The model under review builds one solid part; all positions refer to its coordinate system, in mm. A direction names the side the tool comes from. Coordinates: 2 decimals unless noted, no trailing zeros. Loops run counter-clockwise (first coordinate to the right, second up) from the corner with the lowest first, then second, coordinate; pieces in that order, holes last. Notation, with made-up numbers: (79.5, 5.25) - (90.5, 5.25) arc R29 ccw to (90.5, 26.25) - close; hole circle Ø5 at (5, 50.5). An arc over 180 degrees is marked (long way). Answer in a Markdown table with one row per item. Add a question column.
(1) We need section A-A on y = 26.25. Write out the cut boundary in (x, z), plus the area to 3 significant figures.
(2) For P1, Ø16.5, axis at y = 12, z = -68, coming from the -X side; P2, Ø8, axis at y = 12, z = -49, coming from the -X side; P3, Ø11, axis at x = 110, y = 21.5, coming from the +Z side, all flat-tipped, find the tip position at first contact; note any pin that passes through.
(3) For line 1 along Z through (x, y) = (135, 1.75); line 2 along Z through (x, y) = (95, 3.5); line 3 along X through (y, z) = (0.8, -70), list the stretches that pass through material, from the lowest coordinate up.
(4) We need section D-D on x = 109.5. Write out the cut boundary in (y, z), plus the area to 3 significant figures.
(5) We need section B-B on x = 135. Write out the cut boundary in (y, z), plus the area to 3 significant figures.
(6) Machinability: for faces 5 (the flat face through (12, 15, -49.271)), 6 (the flat face through (86, 10, -13)), 7 (the flat face through (47, 9, -46.789)), which of the approach directions +Z, -Z, +X, -X, +Y, -Y give a long, thin tool a straight path to every point of the face, cutting with its end or side? Answer none if there is none.
(7) Mouldability with a two-part tool opening along X and no side actions: class faces 1 (the flat face through (110, 15, -44.515)), 2 (the flat face through (7.038, 15, -44)), 3 (the flat face through (96.557, 6, -63)), 4 (the flat face through (76.557, 6, -53)) as +X half, -X half, draft (parallel to the pull), parting line (faces both ways), or undercut.
(8) We need section C-C on x = 32.5. Write out the cut boundary in (y, z), plus the area to 3 significant figures.
from build123d import *

# Parameters (mm, degrees)
ESQUISSE1_W      = 140
ESQUISSE1_H      = 75
ESQUISSE1_R      = 2
EXTRUSION1_DEPTH = 3
ESQUISSE2_W      = 45
ESQUISSE2_H      = 45
EXTRUSION2_DEPTH = 15
CONG_1_R         = 2
ESQUISSE3_W      = 10
ESQUISSE3_H      = 10
EXTRUSION3_DEPTH = 25
ESQUISSE4_W      = 25
ESQUISSE4_H      = 10
EXTRUSION4_DEPTH = 20
ESQUISSE5_W      = 20
ESQUISSE5_H      = 5
EXTRUSION5_DEPTH = 7
ESQUISSE6_W      = 10
ESQUISSE6_H      = 15
EXTRUSION6_DEPTH = 25


with BuildPart() as part:
    # Esquisse1 → Extrusion1 (new body)
    with BuildSketch(Plane(origin=(0, 0, 0), x_dir=(1, 0, 0), z_dir=(0, 1, 0))):
        with Locations((70, 37.5)):
            Rectangle(ESQUISSE1_W, ESQUISSE1_H)
        with Locations((5, 70)):
            Circle(ESQUISSE1_R, mode=Mode.SUBTRACT)
        with Locations((135, 70)):
            Circle(ESQUISSE1_R, mode=Mode.SUBTRACT)
        with Locations((135, 5)):
            Circle(ESQUISSE1_R, mode=Mode.SUBTRACT)
        with Locations((5, 5)):
            Circle(ESQUISSE1_R, mode=Mode.SUBTRACT)
    extrude(amount=EXTRUSION1_DEPTH)

    # Esquisse2 → Extrusion2 (add)
    with BuildSketch(Plane(origin=(0, 3, 0), x_dir=(1, 0, 0), z_dir=(0, 1, 0))):
        with Locations((47.129827859, 24.288749044)):
            Rectangle(ESQUISSE2_W, ESQUISSE2_H)
    extrude(amount=EXTRUSION2_DEPTH)

    # Congé1
    cong_1_edges = [part.edges().sort_by_distance(p)[0] for p in [
        (24.629827859, 18, -24.288749044),
        (47.129827859, 18, -1.788749044),
        (69.629827859, 18, -24.288749044),
        (47.129827859, 18, -46.788749044),
    ]]
    fillet(cong_1_edges, radius=CONG_1_R)

    # Esquisse3 → Extrusion3 (add)
    with BuildSketch(Plane(origin=(0, 3, 0), x_dir=(1, 0, 0), z_dir=(0, 1, 0))):
        with Locations((110.370603903, 64.515282671)):
            Rectangle(ESQUISSE3_W, ESQUISSE3_H)
        with Locations((12.038471753, 44.271083815)):
            Rectangle(ESQUISSE3_W, ESQUISSE3_H)
        with Locations((110.370603903, 49.515282671)):
            Rectangle(ESQUISSE3_W, ESQUISSE3_H)
        with Locations((110.370603903, 34.515282671)):
            Rectangle(ESQUISSE3_W, ESQUISSE3_H)
    extrude(amount=EXTRUSION3_DEPTH)

    # Esquisse4 → Extrusion4 (add)
    with BuildSketch(Plane(origin=(0, 3, 0), x_dir=(1, 0, 0), z_dir=(0, 1, 0))):
        with Locations((43.077660713, 67.06403932)):
            Rectangle(ESQUISSE4_W, ESQUISSE4_H)
        with Locations((43.077660713, 54.56403932)):
            Rectangle(ESQUISSE4_W, ESQUISSE4_H)
    extrude(amount=EXTRUSION4_DEPTH)

    # Esquisse5 → Extrusion5 (add)
    with BuildSketch(Plane(origin=(0, 3, 0), x_dir=(1, 0, 0), z_dir=(0, 1, 0))):
        with Locations((86.557419786, 62.697517929)):
            Rectangle(ESQUISSE5_W, ESQUISSE5_H)
        with Locations((86.557419786, 52.697517929)):
            Rectangle(ESQUISSE5_W, ESQUISSE5_H)
        with Locations((86.557419786, 42.697517929)):
            Rectangle(ESQUISSE5_W, ESQUISSE5_H)
        with Locations((86.557419786, 32.697517929)):
            Rectangle(ESQUISSE5_W, ESQUISSE5_H)
        with Locations((86.557419786, 22.697517929)):
            Rectangle(ESQUISSE5_W, ESQUISSE5_H)
        with Locations((86.557419786, 12.697517929)):
            Rectangle(ESQUISSE5_W, ESQUISSE5_H)
    extrude(amount=EXTRUSION5_DEPTH)

    # Esquisse6 → Extrusion6 (add)
    with BuildSketch(Plane(origin=(0, 3, 0), x_dir=(1, 0, 0), z_dir=(0, 1, 0))):
        with Locations((15.904188898, 68.024450773)):
            Rectangle(ESQUISSE6_W, ESQUISSE6_H)
    extrude(amount=EXTRUSION6_DEPTH)


solid = part.part
Outcome:
| question | item | result |
|---|---|---|
| 1 | outline | (7.04, -49.27) - (17.04, -49.27) - (17.04, -39.27) - (7.04, -39.27) - close; (10.9, -75.52) - (20.9, -75.52) - (20.9, -60.52) - (10.9, -60.52) - close; (105.37, -69.52) - (115.37, -69.52) - (115.37, -59.52) - (105.37, -59.52) - close; (105.37, -54.52) - (115.37, -54.52) - (115.37, -44.52) - (105.37, -44.52) - close; (105.37, -39.52) - (115.37, -39.52) - (115.37, -29.52) - (105.37, -29.52) - close |
| 1 | area | 550 mm² |
| 2 | P1 | x = 10.9 |
| 2 | P2 | x = 7.04 |
| 2 | P3 | z = -29.52 |
| 3 | line 1 | -75 to -72, -68 to -7, -3 to 0 |
| 3 | line 2 | -65.2 to -60.2, -55.2 to -50.2, -45.2 to -40.2, -35.2 to -30.2, -25.2 to -20.2, -15.2 to -10.2 |
| 3 | line 3 | 0 to 3, 7 to 133, 137 to 140 |
| 4 | outline | (0, -75) - (3, -75) - (3, -69.52) - (28, -69.52) - (28, -59.52) - (3, -59.52) - (3, -54.52) - (28, -54.52) - (28, -44.52) - (3, -44.52) - (3, -39.52) - (28, -39.52) - (28, -29.52) - (3, -29.52) - (3, 0) - (0, 0) - close |
| 4 | area | 975 mm² |
| 5 | outline | (0, -75) - (3, -75) - (3, -72) - (0, -72) - close; (0, -68) - (3, -68) - (3, -7) - (0, -7) - close; (0, -3) - (3, -3) - (3, 0) - (0, 0) - close |
| 5 | area | 201 mm² |
| 6 | face 5 | -X, +Y |
| 6 | face 6 | +Z, -Z, +X, +Y |
| 6 | face 7 | +Y |
| 7 | face 1 | draft |
| 7 | face 2 | -X half |
| 7 | face 3 | undercut |
| 7 | face 4 | undercut |
| 8 | outline | (0, -75) - (3, -75) - (3, -72.06) - (23, -72.06) - (23, -62.06) - (3, -62.06) - (3, -59.56) - (23, -59.56) - (23, -49.56) - (3, -49.56) - (3, -46.79) - (16, -46.79) arc R2 ccw to (18, -44.79) - (18, -3.79) arc R2 ccw to (16, -1.79) - (3, -1.79) - (3, 0) - (0, 0) - close |
| 8 | area | 1,300 mm² |
